Geometry check sheet. Reference: the model listing, model coordinates, mm. Face numbers are marked on the shaded views. A direction names the side the tool comes from. Round coordinates to 2 decimals unless told otherwise and drop trailing zeros. Order: outer loops, then holes, each group sorted by start corner. A loop starts at its lowest first (then second) coordinate and runs counter-clockwise, first axis right, second up.
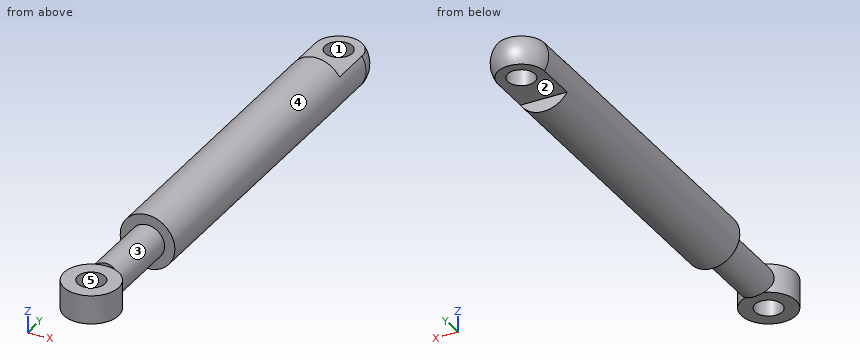
```python
from build123d import *

# Parameters (mm, degrees)
CUT_EXTRUDE1_DEPTH      = 56.290143787
CUT_EXTRUDE1_DEPTH_BACK = 56.290143787
SKETCH4_3_R             = 4
SKETCH4_4_R             = 4
BOSS_EXTRUDE1_DEPTH     = 2.1
CUT_EXTRUDE2_DEPTH      = 56.290143794
CUT_EXTRUDE3_DEPTH      = 56.290143794
CUT_EXTRUDE3_DEPTH_BACK = 56.290143794
SKETCH1_R               = 2


with BuildPart() as part:
    # Sketch3 → Revolve2 (revolve)
    with BuildSketch(Plane.XY, mode=Mode.PRIVATE) as revolve2_sk:
        with BuildLine():
            Line((0, 0), (4, 0))
            Line((4, 0), (4, 51))
            ThreePointArc((4, 51), (2.828427125, 53.828427125), (0, 55))
            Line((0, 55), (0, 0))
        make_face()
    revolve(revolve2_sk.sketch.rotate(Axis((0, 0, 0), (0, 1, 0)), 90), axis=Axis((0, 0, 0), (0, 1, 0)))

    # Sketch4 → Revolve3 (revolve)
    with BuildSketch(Plane.XY):
        with BuildLine():
            Line((2.5, -11.877501001), (2.5, 0))
            Line((2.5, 0), (0, 0))
            Line((0, 0), (0, -11))
            ThreePointArc((0, -11), (1.324764885, -11.225745372), (2.5, -11.877501001))
        make_face()
    revolve(axis=Axis((0, 0, 0), (0, -1, 0)))

    # Sketch4_3 → Cut-Extrude1 (cut, two sides: drawn at the far end of the back side and taken through both)
    with BuildSketch(Plane.XY.offset(-CUT_EXTRUDE1_DEPTH_BACK)):
        with Locations((0, -15)):
            Circle(SKETCH4_3_R)
    extrude(amount=CUT_EXTRUDE1_DEPTH + CUT_EXTRUDE1_DEPTH_BACK, mode=Mode.SUBTRACT)

    # Sketch4_4 → Boss-Extrude1 (add, symmetric)
    with BuildSketch(Plane.XY):
        with Locations((0, -15)):
            Circle(SKETCH4_4_R)
    extrude(amount=BOSS_EXTRUDE1_DEPTH, both=True)

    # Sketch5 → Cut-Extrude2 (cut, symmetric)
    with BuildSketch(Plane(origin=(0, 0, 0), x_dir=(0, 0, -1), z_dir=(1, 0, 0))):
        Polygon((-2.1, 211.719272535), (-2.1, 54.404408906), (-2.1, 45), (-4, 45), (-161.314863629, 45), (-388.853749338, 262.296849414), (-229.638885709, 429.016121949), align=None)
    cut_extrude2 = extrude(amount=CUT_EXTRUDE2_DEPTH, both=True, mode=Mode.SUBTRACT)

    # Mirror1: Cut-Extrude2 across plane
    add(cut_extrude2.mirror(Plane.XY), mode=Mode.SUBTRACT)

    # Sketch1 → Cut-Extrude3 (cut, two sides: drawn at the far end of the back side and taken through both)
    with BuildSketch(Plane.XY.offset(-CUT_EXTRUDE3_DEPTH_BACK)):
        with Locations(Location((0, 51, 0), (0, 0, 90))):
            Circle(SKETCH1_R)
        with Locations((0, -15)):
            Circle(SKETCH1_R)
    extrude(amount=CUT_EXTRUDE3_DEPTH + CUT_EXTRUDE3_DEPTH_BACK, mode=Mode.SUBTRACT)


solid = part.part
```
(1) Sectioned sample at C-C, the plane y = 37.5. Record the cut outline in (x, z), and give its area (3 significant figures).
Returned:
outline: circle Ø8 at (0, 0)
area: 50.3 mm2
(2) Sectioned sample at B-B, the plane z = 0.75. Record the cut outline in (x, y), and give its area (3 significant figures).
Returned:
outline: (-3.93, 0) - (-2.38, 0) - (-2.38, -11.79) arc R4 ccw (long way) to (2.38, -11.79) - (2.38, 0) - (3.93, 0) - (3.93, 51) arc R3.93 ccw to (-3.93, 51) - close; hole circle Ø4 at (0, -15); hole circle Ø4 at (0, 51)
area: 504 mm2
(3) Set-up check for the marked faces 3, 4 and 5: record each of +Z, -Z, +X, -X, +Y, -Y from which the full face is reachable in a straight line by a thin tool's end or side.
Returned:
face 3: none
face 4: +Y
face 5: +Z, -Z
(4) Depth check by flat-ended pin: P1, Ø2.5, axis at x = 0, y = -15, coming from the -Z side; P2, Ø1, axis at x = -0.5, z = 2, coming from the +Y side; P3, Ø1.5, axis at x = -0.5, y = 18, coming from the -Z side; P4, Ø1.5, axis at x = 1.5, z = -3, coming from the +Y side. Enter the tip coordinate at first touch or a pass-through.
Returned:
P1: passes through
P2: stops at y = 54.68
P3: stops at z = -4
P4: stops at y = 45
(5) Sectioned sample at A-A, the plane y = -15. Record the cut outline in (x, z), and give its area (3 significant figures).
Returned:
outline: (-4, -2.1) - (-2, -2.1) - (-2, 2.1) - (-4, 2.1) - close; (2, -2.1) - (4, -2.1) - (4, 2.1) - (2, 2.1) - close
area: 16.8 mm2
(6) Draft check along Y on the marked faces 1 and 2. Enter one of: released by +Y, released by -Y, zero draft, split by the parting line, or undercut.
Returned:
face 1: undercut
face 2: zero draft
(7) Material ranges on line 1 (X direction, y = -15, z = 0.55); line 2 (Y direction, x = 0.25, z = 3.75); line 3 (X direction, y = -10, z = 0), recorded low to high.
Returned:
line 1: x = -4 to -2, 2 to 4
line 2: y = 0 to 45
line 3: x = -2.5 to 2.5
